from build123d import *

# Parameters (mm, degrees)
SKETCH_1_R          = 4.25
EXTRUDE_1_DEPTH     = 320
SKETCH_2_R          = 3.5
CUT_EXTRUDE_1_DEPTH = 494
SKETCH_3_R          = 3.5
SKETCH_3_R_2        = 2.5
EXTRUDE_2_DEPTH     = 40


with BuildPart() as part:
    # 草图1 → 凸台-拉伸1 (new body)
    with BuildSketch(Plane(origin=(0, 0, 0), x_dir=(1, 0, 0), z_dir=(0, 1, 0))):
        Circle(SKETCH_1_R)
    extrude(amount=EXTRUDE_1_DEPTH)

    # 草图2 → 切除-拉伸1 (cut)
    with BuildSketch(Plane(origin=(0, 0, 0), x_dir=(1, 0, 0), z_dir=(0, 1, 0))):
        Circle(SKETCH_2_R)
    extrude(amount=CUT_EXTRUDE_1_DEPTH, mode=Mode.SUBTRACT)

    # 草图3 → 凸台-拉伸2 (add, symmetric)
    with BuildSketch(Plane(origin=(0, 0, 0), x_dir=(1, 0, 0), z_dir=(0, 1, 0))):
        Circle(SKETCH_3_R)
        Circle(SKETCH_3_R_2, mode=Mode.SUBTRACT)
    extrude(amount=EXTRUDE_2_DEPTH, both=True)


solid = part.part
Work out the finished part from the listing and answer in its coordinate system (mm). A direction names the side the tool comes from. Coordinates: 2 decimals unless noted, no trailing zeros. Order: outer loops, then holes, each group sorted by start corner. A loop starts at its lowest first (then second) coordinate and runs counter-clockwise, first axis right, second up. Notation, with made-up numbers: (51, 36.25) - (64, 36.25) arc R11 ccw to (64, 52.25) - close; hole circle Ø9 at (-14, 56.5). An arc over 180 degrees is marked (long way). Put each result on its own line as item: value. Start each with the question number.
1) Flat-ended cylindrical pins translate along their axes: pin 1 (2 mm diameter, centred on x = 0, z = 1, fed in from +Y); pin 2 (3 mm diameter, centred on x = -2.5, y = 97, fed in from -Z). Find the tip coordinate at first contact, or state that the pin passes through.
2) For faces 4 (the flat face through (2, 40, 2)), 5 (the cylindrical face through (2.285, 157.76, -3.584)), determine the directions among +Z, -Z, +X, -X, +Y, -Y from which every point of the face is accessible in a straight line to the end or side of a thin tool.
3) Find section D-D (y = 136.5). Give the vertices of the cut face in (x, z), plus the area to 3 significant figures.
4) Find section C-C (y = -7). Give the vertices of the cut face in (x, z).
5) Find the intervals of material crossed by line 1 (Z direction, x = 0, y = 23); line 2 (Z direction, x = 0, y = 113), in increasing order. Write a range as from..to.
6) Find section A-A (z = 0). Give the vertices of the cut face in (x, y), plus the area to 3 significant figures.
7) Find section B-B (x = 0). Give the vertices of the cut face in (y, z).
8) For a pull along Z with two mould halves and no side action, classify faces 1 (the flat face through (2, -40, 2)), 2 (the cylindrical face through (3.233, 178.04, 1.341)), 3 (the cylindrical face through (3.233, -19.72, 1.341)) as released by +Z, released by -Z, zero draft, split by the parting line, or undercut.
Results list:
1. pin 1: passes through
1. pin 2: stops at z = -4.13
2. face 4: +Y
2. face 5: +Y, -Y
3. outline: circle Ø8.5 at (0, 0); hole circle Ø7 at (0, 0)
3. area: 18.3 mm^2
4. outline: circle Ø7 at (0, 0); hole circle Ø5 at (0, 0)
5. line 1: z = -4.25..-2.5, 2.5..4.25
5. line 2: z = -4.25..-3.5, 3.5..4.25
6. outline: (-4.25, 0) - (-3.5, 0) - (-3.5, -40) - (-2.5, -40) - (-2.5, 40) - (-3.5, 40) - (-3.5, 320) - (-4.25, 320) - close; (2.5, -40) - (3.5, -40) - (3.5, 0) - (4.25, 0) - (4.25, 320) - (3.5, 320) - (3.5, 40) - (2.5, 40) - close
6. area: 640 mm^2
7. outline: (-40, -3.5) - (0, -3.5) - (0, -4.25) - (320, -4.25) - (320, -3.5) - (40, -3.5) - (40, -2.5) - (-40, -2.5) - close; (-40, 2.5) - (40, 2.5) - (40, 3.5) - (320, 3.5) - (320, 4.25) - (0, 4.25) - (0, 3.5) - (-40, 3.5) - close
8. face 1: zero draft
8. face 2: undercut
8. face 3: split by the parting line
